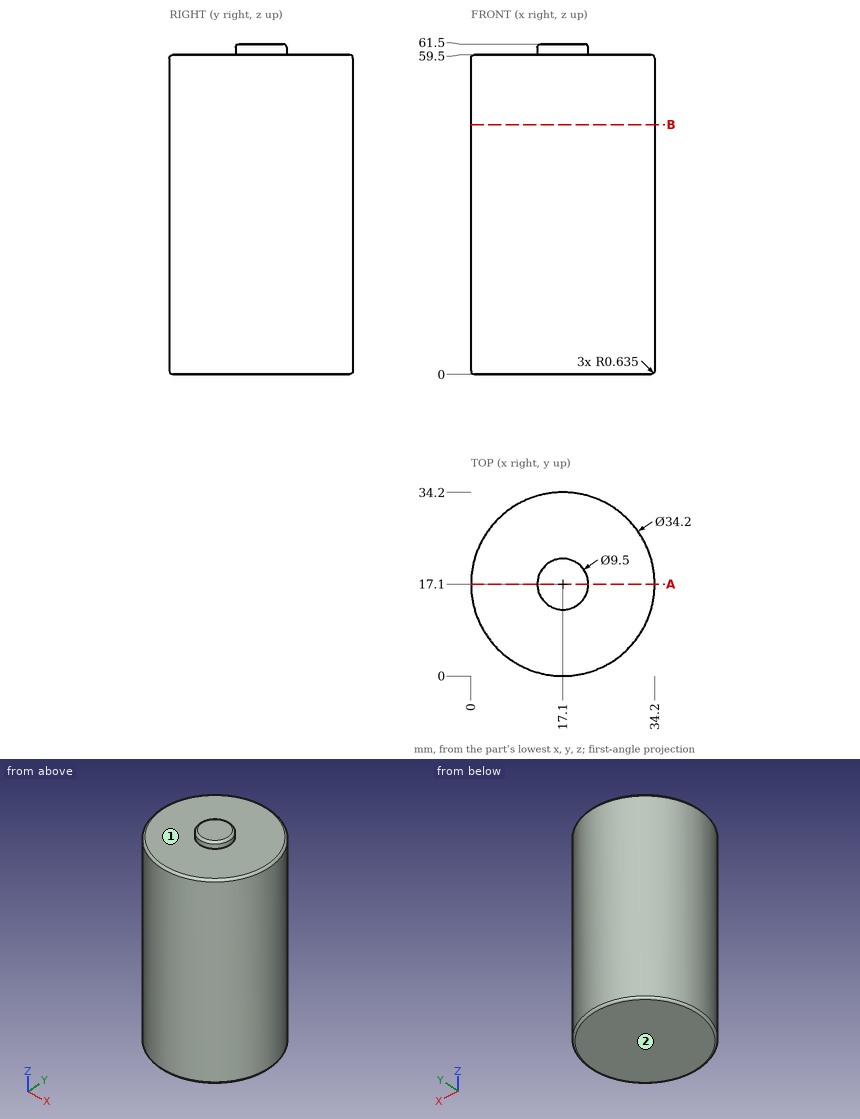
Answer from the drawing. Dimensions are ordinates in mm from the lowest x, y and z of the part. A direction names the side the tool comes from. Round coordinates to 2 decimals unless told otherwise and drop trailing zeros. Loops run counter-clockwise (first coordinate to the right, second up) from the corner with the lowest first, then second, coordinate; pieces in that order, holes last.
Q1. Each of these flat-tipped pins is pushed along its axis until it touches: pin 1 (1.5 mm diameter, centred on x = 13, z = 35.5, fed in from +Y); pin 2 (1.5 mm diameter, centred on x = 27.5, z = 52, fed in from +Y); pin 3 (1 mm diameter, centred on x = 23, y = 27, fed in from -Z); pin 4 (1 mm diameter, centred on x = 5, z = 53, fed in from -Y). Where does it stop, or does it pass through?
Q2. Section A-A on y = 17.1 is taken. Write down the section's boundary in (x, z) (3 decimals).
Q3. Consider probe 1 along Z at (x, y) = (24.5, 20); probe 2 along X at (y, z) = (3.5, 56); probe 3 along X at (y, z) = (27.5, 19.5). Determine where each line is inside the solid, lowest interval first.
Q4. Section B-B on z = 46.5 is taken. Write down the section's boundary in (x, y).
Q5. Which of the six approach directions +Z, -Z, +X, -X, +Y, -Y give full straight-line access (tool end or side, diameter ignored) to the marked faces 1 and 2?
Output:
1. pin 1: stops at y = 33.87
1. pin 2: stops at y = 31.22
1. pin 3: stops at z = 0
1. pin 4: stops at y = 4.54
2. outline: (0, 0.635) arc R0.635 ccw to (0.635, 0) - (33.565, 0) arc R0.635 ccw to (34.2, 0.635) - (34.2, 58.865) arc R0.635 ccw to (33.565, 59.5) - (21.85, 59.5) - (21.85, 60.865) arc R0.635 ccw to (21.215, 61.5) - (12.985, 61.5) arc R0.635 ccw to (12.35, 60.865) - (12.35, 59.5) - (0.635, 59.5) arc R0.635 ccw to (0, 58.865) - close
3. probe 1: z = 0 to 59.5
3. probe 2: x = 6.73 to 27.47
3. probe 3: x = 3.53 to 30.67
4. outline: circle Ø34.2 at (17.1, 17.1)
5. face 1: +Z
5. face 2: -Z, +X, -X, +Y, -Y
